Can you work these out from the model? Positions are in its coordinate system, mm. A direction names the side the tool comes from. Coordinates: 2 decimals unless noted, no trailing zeros. Order: outer loops, then holes, each group sorted by start corner. A loop starts at its lowest first (then second) coordinate and runs counter-clockwise, first axis right, second up. Notation, with made-up numbers: (-22.75, -26) -> (31.25, -26) arc R34 cw to (31.25, 10) -> close; hole circle Ø1 at (-39.75, 65.25). An arc over 180 degrees is marked (long way). Use a Markdown table: item, result. Add a question column.
1. If I drill on line 1 along Y through (x, z) = (19, 0); line 2 along X through (y, z) = (-57.5, -15); line 3 along X through (y, z) = (-50.5, -14), over which ranges is the centre line in solid material (lowest first)? Write a range as from..to.
2. Suppose I cut it at A-A, the plane x = -5. List the corners of the cut face in (y, z) for me, then the cut area to 3 significant figures.
3. For pin 1 Ø5.5 at (x, z) = (-14, -6.5) entering from +Y; pin 2 Ø6 at (x, y) = (17, 37) entering from -Z; pin 3 Ø16.5 at (x, z) = (-5.5, -0.5) entering from -Y, each with a flat end and sliding along its axis, tell me the tip position at first contact or that it passes through.
4. Suppose I cut it at B-B, the plane y = 0. List the corners of the cut face in (x, z) for me, then the cut area to 3 significant figures.
5. For faces 4 (the flat face through (-9, 25, 0)), 5 (the cylindrical face through (-23.196, 0.266, 23.289)), 6 (the flat face through (0, 1, -27)), 7 (the flat face through (6.35, 47, 24)), which set-ups out of +Z, -Z, +X, -X, +Y, -Y let a thin tool reach every point of the face, with its end or its side?
6. We'd pull the mould along Y, two halves only. Please class faces 1 (the cylindrical face through (-23.196, -23.289, 0.266)), 2 (the cylindrical face through (-9.633, 23.289, 23.196)), 3 (the cylindrical face through (4.639, 0.231, -24.304)): pulls with the +Y half, pulls with the -Y half, needs draft (parallel to the pull), parting line crosses it, or undercut.
7. Suppose I cut it at D-D, the plane x = 3. List the corners of the cut face in (y, z) for me.
```python
from build123d import *

# Parameters (mm, degrees)
SKETCH1_R           = 63.5
BOSS_EXTRUDE1_DEPTH = 6.35
SKETCH2_R           = 52.5
SKETCH2_R_2         = 50.00625
BOSS_EXTRUDE2_DEPTH = 19.05
SKETCH3_W           = 50
SKETCH3_H           = 50
BOSS_EXTRUDE3_DEPTH = 25
SKETCH4_W           = 45
SKETCH4_H           = 45
CUT_EXTRUDE1_DEPTH  = 26.35
FILLET1_R           = 6


with BuildPart() as part:
    # Sketch1 → Boss-Extrude1 (new body)
    with BuildSketch(Plane(origin=(0, 0, 0), x_dir=(0, 0, -1), z_dir=(1, 0, 0))):
        Circle(SKETCH1_R)
    extrude(amount=BOSS_EXTRUDE1_DEPTH)

    # Sketch2 → Boss-Extrude2 (add)
    with BuildSketch(Plane(origin=(6.35, 0, 0), x_dir=(0, 0, -1), z_dir=(1, 0, 0))):
        with Locations(Location((0, 0, 0), (0, 0, 180))):
            Circle(SKETCH2_R)
        with Locations(Location((0, 0, 0), (0, 0, 180))):
            Circle(SKETCH2_R_2, mode=Mode.SUBTRACT)
    extrude(amount=BOSS_EXTRUDE2_DEPTH)

    # Sketch3 → Boss-Extrude3 (add)
    with BuildSketch(Plane.ZY):
        Rectangle(SKETCH3_W, SKETCH3_H)
    extrude(amount=BOSS_EXTRUDE3_DEPTH)

    # Sketch4 → Cut-Extrude1 (cut)
    with BuildSketch(Plane(origin=(6.35, 0, 0), x_dir=(0, 0, -1), z_dir=(1, 0, 0))):
        Rectangle(SKETCH4_W, SKETCH4_H)
    extrude(amount=-CUT_EXTRUDE1_DEPTH, mode=Mode.SUBTRACT)

    # Fillet1
    fillet1_edges = [part.edges().sort_by_distance(p)[0] for p in [
        (-12.5, -25, 25),
        (-12.5, 25, 25),
        (-12.5, 25, -25),
        (-12.5, -25, -25),
        (-25, 0, 25),
        (-25, 25, 0),
        (-25, 0, -25),
        (-25, -25, 0),
        (6.35, 0, -22.5),
        (6.35, 22.5, 0),
        (6.35, 0, 22.5),
        (6.35, -22.5, 0),
        (-6.825, 22.5, 22.5),
        (-6.825, -22.5, 22.5),
        (-6.825, -22.5, -22.5),
        (-6.825, 22.5, -22.5),
    ]]
    fillet(fillet1_edges, radius=FILLET1_R)


solid = part.part
```
Worked out:
| question | item | result |
|---|---|---|
| 1 | line 1 | y = -52.5..-50.01, 50.01..52.5 |
| 1 | line 2 | x = 0..6.35 |
| 1 | line 3 | x = 0..25.4 |
| 2 | outline | (-25, -19) arc R6 ccw to (-19, -25) -> (19, -25) arc R6 ccw to (25, -19) -> (25, 19) arc R6 ccw to (19, 25) -> (-19, 25) arc R6 ccw to (-25, 19) -> close; hole (-22.5, -16.5) arc R6 ccw to (-16.5, -22.5) -> (16.5, -22.5) arc R6 ccw to (22.5, -16.5) -> (22.5, 16.5) arc R6 ccw to (16.5, 22.5) -> (-16.5, 22.5) arc R6 ccw to (-22.5, 16.5) -> close |
| 2 | area | 475 mm² |
| 3 | pin 1 | stops at y = 25 |
| 3 | pin 2 | stops at z = -40 |
| 3 | pin 3 | stops at y = -63.5 |
| 4 | outline | (-25, -19) arc R6 ccw to (-19, -25) -> (0, -25) -> (0, -63.5) -> (6.35, -63.5) -> (6.35, -52.5) -> (25.4, -52.5) -> (25.4, -50.01) -> (6.35, -50.01) -> (6.35, -28.5) arc R6 ccw to (0.35, -22.5) -> (-20, -22.5) -> (-20, 22.5) -> (0.35, 22.5) arc R6 ccw to (6.35, 28.5) -> (6.35, 50.01) -> (25.4, 50.01) -> (25.4, 52.5) -> (6.35, 52.5) -> (6.35, 63.5) -> (0, 63.5) -> (0, 25) -> (-19, 25) arc R6 ccw to (-25, 19) -> close |
| 4 | area | 935 mm² |
| 5 | face 4 | +Z, -Z, -X, +Y |
| 5 | face 5 | +Z, -X, +Y, -Y |
| 5 | face 6 | -X |
| 5 | face 7 | +X |
| 6 | face 1 | pulls with the -Y half |
| 6 | face 2 | pulls with the +Y half |
| 6 | face 3 | undercut |
| 7 | outline | circle Ø127 at (0, 0); hole (-23.12, -16.5) arc R6.62 ccw to (-16.5, -23.12) -> (16.5, -23.12) arc R6.62 ccw to (23.12, -16.5) -> (23.12, 16.5) arc R6.62 ccw to (16.5, 23.12) -> (-16.5, 23.12) arc R6.62 ccw to (-23.12, 16.5) -> close |
